Build history of the part. All positions in model axes, mm. Face numbers are marked on the shaded views. A direction names the side the tool comes from. Give positions to 0.01 mm unless a question says otherwise; leave off trailing zeros. Write each loop counter-clockwise with the first axis right and the second up, starting at its lowest first coordinate (ties: lowest second). Pieces come first, ordered by that corner, then holes.
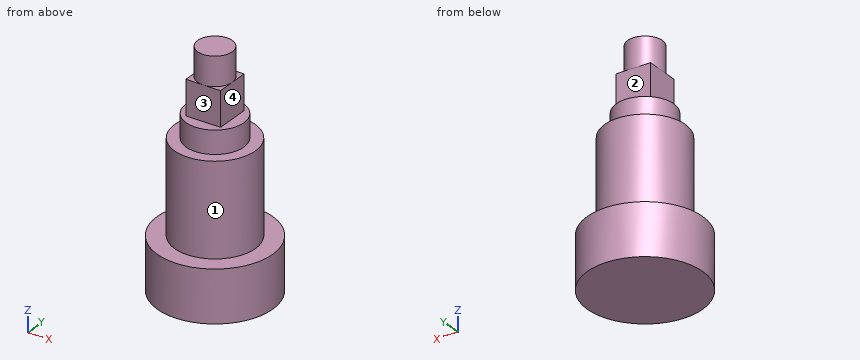
Autodesk Inventor part; units mm, degrees
ref_plane "YZ Plane" through (0, 0, 0) normal (1, 0, 0) x (0, 1, 0)
ref_plane "XZ Plane" through (0, 0, 0) normal (0, 1, 0) x (-1, 0, 0)
ref_plane "XY Plane" through (0, 0, 0) normal (0, 0, 1) x (1, 0, 0)
sketch "Sketch1" plane through (0, 0, 0) normal (0, 0, 1) x (1, 0, 0)
  circle A0 centre (0, 0) radius 5
  dimension "d0" = 10
extrude "Extrusion1" add sketch "Sketch1" along normal blind 4.5
sketch "Sketch2" plane through (0, 0, 4.5) normal (0, 0, 1) x (1, 0, 0)
  circle A0 centre (0, 0) radius 5
  circle A1 centre (0, 0) radius 3.5
  dimension "d3" = 7
extrude "Extrusion2" add sketch "Sketch2" along normal blind 8 contours A1
sketch "Sketch3" plane through (0, 0, 12.5) normal (0, 0, 1) x (1, 0, 0)
  circle A0 centre (0, 0) radius 5
  circle A1 centre (0, 0) radius 2.5
  dimension "d6" = 5
extrude "Extrusion3" add sketch "Sketch3" along normal blind 2 contours A1
sketch "Sketch4" plane through (0, 0, 14.5) normal (0, 0, 1) x (1, 0, 0)
  circle A0 centre (0, 0) radius 2.5
  line L0 (-1.5, 1.5) -> (1.5, 1.5)
  line L1 (1.5, 1.5) -> (1.5, -1.5)
  line L2 (1.5, -1.5) -> (-1.5, -1.5)
  line L3 (-1.5, -1.5) -> (-1.5, 1.5)
  line L4 (-1.5, 1.5) -> (1.5, -1.5) construction
  line L5 (1.5, 1.5) -> (-1.5, -1.5) construction
  dimension "d9" = 3
  dimension "d10" = 3
extrude "Extrusion4" add sketch "Sketch4" along normal blind 3 contours L0 L1 L2 L3
sketch "Sketch5" plane through (0, 0, 17.5) normal (0, 0, 1) x (1, 0, 0)
  circle A0 centre (0, 0) radius 1.5
  dimension "d13" = 3
extrude "Extrusion5" add sketch "Sketch5" along normal blind 2.5
thread "Thread1"
properties part number "24 - Valve Disc Spindle" material "Bronze, Soft Tin"
(1) Saw through at A-A, the plane y = -0.75. List the corners of the cut face in (x, z), plus the area to 3 significant figures.
(2) Probe line 1 (Z direction, x = 2.75, y = -2.5); line 2 (Z direction, x = -2.5, y = -1.25); line 3 (X direction, y = 0.75, z = 17.25). List the from-to ranges inside material, lowest first.
(3) Saw through at B-B, the plane x = 3.25. List the corners of the cut face in (y, z), plus the area to 3 significant figures.
(4) Drop flat-ended pins along their axis: pin 1 (5 mm diameter, centred on x = -3.5, z = 3, fed in from -Y); pin 2 (1.5 mm diameter, centred on y = 0, z = 16, fed in from +X); pin 3 (3.5 mm diameter, centred on x = -0.5, z = 15.5, fed in from +Y). Give the stop position or say it passes through.
(5) Saw through at C-C, the plane z = 7.5. List the corners of the cut face in (x, y), plus the area to 3 significant figures.
(6) 3-axis set-ups, long thin cutter, end or side, ignore diameter. For the marked faces 1, 2, 3 and 4: which of +Z, -Z, +X, -X, +Y, -Y reach the whole face in a straight line?
Computed values:
1. outline: (-4.94, 0) - (4.94, 0) - (4.94, 4.5) - (3.42, 4.5) - (3.42, 12.5) - (2.38, 12.5) - (2.38, 14.5) - (1.5, 14.5) - (1.5, 17.5) - (1.3, 17.5) - (1.3, 20) - (-1.3, 20) - (-1.3, 17.5) - (-1.5, 17.5) - (-1.5, 14.5) - (-2.38, 14.5) - (-2.38, 12.5) - (-3.42, 12.5) - (-3.42, 4.5) - (-4.94, 4.5) - close
1. area: 124 mm2
2. line 1: z = 0 to 4.5
2. line 2: z = 0 to 12.5
2. line 3: x = -1.5 to 1.5
3. outline: (-3.8, 0) - (3.8, 0) - (3.8, 4.5) - (1.3, 4.5) - (1.3, 12.5) - (-1.3, 12.5) - (-1.3, 4.5) - (-3.8, 4.5) - close
3. area: 55.0 mm2
4. pin 1: stops at y = -4.9
4. pin 2: stops at x = 1.5
4. pin 3: stops at y = 2.5
5. outline: circle Ø7 at (0, 0)
5. area: 38.5 mm2
6. face 1: +Z
6. face 2: +Z, +X, -X, +Y
6. face 3: +Z, +X, -X, -Y
6. face 4: +Z, +X, +Y, -Y
